Input: part model. Units: mm. Frame: model coordinates. A direction names the side the tool comes from. Round coordinates to 2 decimals unless told otherwise and drop trailing zeros. Loops run counter-clockwise (first coordinate to the right, second up) from the corner with the lowest first, then second, coordinate; pieces in that order, holes last. Notation, with made-up numbers: M 49.25,-5 L 98.25,-5 A21 ccw 98.25,11 Z; hole C 79,66.5 d1. An arc over 180 degrees is marked long. Use one line per item in the form item = value. Start each with the question number.
Q1. First-contact query: P1, Ø0.6, axis at x = 0, z = -7.5, coming from the +Y side; P2, Ø0.7, axis at y = -3.5, z = -5, coming from the -X side. Flat tips, straight axial feed; report the tip coordinate or a pass-through.
Q2. Ray query, line 1 along Y through (x, z) = (-0.45, -6.5); line 2 along Y through (x, z) = (0, -8); line 3 along Z through (x, y) = (0.05, 1.25). Return the intervals inside material, ascending.
Q3. Mould query, pull axis Y, two halves, no side actions, for faces 4 (the flat face through (0, -3, -4)), 5 (the flat face through (0.55, 3.5, -3.5)), 6 (the flat face through (0, 4.1, -4)). Classes: pulls with the +Y half, pulls with the -Y half, needs draft (parallel to the pull), parting line crosses it, or undercut.
Q4. Section query D-D, the plane y = 1.5. Output: boundary loops of the cut face in (x, z), and give its area (3 significant figures).
Q5. Section query A-A, the plane z = -1.5. Output: boundary loops of the cut face in (x, y).
Q6. Access query for faces 1 (the flat face through (-0.008, 3.694, -0.641)), 2 (the flat face through (-0.55, 3.5, -3.5)), 3 (the flat face through (0.55, -3.5, -3.5)). Directions: +Z, -Z, +X, -X, +Y, -Y. A direction counts if a zero-diameter tool reaches every point of the face in a straight line with its end or side. Return the directions, or none.
Q7. Section query B-B, the plane z = -6. Output: boundary loops of the cut face in (x, y), and give its area (3 significant figures).
```python
from build123d import *

# Parameters (mm, degrees)
F0_W         = 1.1
F0_H         = 7
F1_DEPTH     = 0.55
F2_W         = 0.7
F2_H         = 0.7
F3_DEPTH     = 1.2
F4_R         = 0.1
F7_DEPTH     = 0.45
F8_W         = 0.8
F8_H         = 0.8
F9_DEPTH     = 3
F10_R        = 0.1
F11_T1_DEPTH = 7.6228122918


# Not quite as in the source:
# - a fillet or chamfer that OpenCascade refuses, or shapes differently, is made with other operations: its cross-section is extruded or revolved along the edge and cut away or added


with BuildPart() as f1:
    # F0 (on Right) → F1 (new body, symmetric)
    with BuildSketch(Plane.YZ):
        with Locations((3.55, -3.5)):
            Rectangle(F0_W, F0_H)
    extrude(amount=F1_DEPTH, both=True)

    # F2 (on face) → F3 (join)
    with BuildSketch(Plane(origin=(0, 0, -7), x_dir=(1, 0, 0), z_dir=(0, 0, -1))):
        with Locations((0, -3.55)):
            Rectangle(F2_W, F2_H)
    extrude(amount=F3_DEPTH)

    # F4
    f4_edges = [f1.edges().sort_by_distance(p)[0] for p in [
        (0.55, 4.1, -3.5),
        (0.55, 3, -3.5),
        (-0.55, 4.1, -3.5),
        (0.35, 3.9, -7.6),
        (-0.35, 3.9, -7.6),
        (0.35, 3.2, -7.6),
        (-0.35, 3.2, -7.6),
        (-0.55, 3, -3.5),
    ]]
    fillet(f4_edges, radius=F4_R)

    # F6 (on mid) → F7 (join, symmetric)
    with BuildSketch(Plane(origin=(0, 3.55, 0), x_dir=(-1, 0, 0), z_dir=(0, 1, 0))):
        with BuildLine():
            ThreePointArc((0.4914213562, -8.1414213562), (0.4265366865, -8.1847759065), (0.35, -8.2))
            Line((0.35, -8.2), (-0.35, -8.2))
            ThreePointArc((-0.35, -8.2), (-0.4265366865, -8.1847759065), (-0.4914213562, -8.1414213562))
            Line((-0.4914213562, -8.1414213562), (-0.6328427125, -8))
            Line((-0.6328427125, -8), (-0.9863961031, -8.3535533906))
            Line((-0.9863961031, -8.3535533906), (-0.8449747468, -8.4949747468))
            ThreePointArc((-0.8449747468, -8.4949747468), (-0.6178784027, -8.6467156728), (-0.35, -8.7))
            Line((-0.35, -8.7), (0.35, -8.7))
            ThreePointArc((0.35, -8.7), (0.6178784027, -8.6467156728), (0.8449747468, -8.4949747468))
            Line((0.8449747468, -8.4949747468), (0.9863961031, -8.3535533906))
            Line((0.9863961031, -8.3535533906), (0.6328427125, -8))
            Line((0.6328427125, -8), (0.4914213562, -8.1414213562))
        make_face()
    extrude(amount=F7_DEPTH, both=True)

    # F8 (on face) → F9 (join, through all)
    with BuildSketch(Plane.XZ.offset(-3)):
        with Locations((0, -5.8)):
            Rectangle(F8_W, F8_H)
    extrude(amount=F9_DEPTH)

    # F10
    f10_edges = [f1.edges().sort_by_distance(p)[0] for p in [
        (-0.4, 1.5, -5.4),
        (-0.4, 1.5, -6.2),
        (0.4, 1.5, -6.2),
        (0.4, 1.5, -5.4),
    ]]
    fillet(f10_edges, radius=F10_R)

    # F11: chamfer of 0.8 x 1.3 on 1 edges, made by hand

    # F11_s2 → F11_t1 (cut)
    with BuildSketch(Plane.YZ.offset(-3.8114061459)):
        Polygon((3.3, 0), (4.1, -1.3), (4.1, 0), align=None)
    extrude(amount=F11_T1_DEPTH, mode=Mode.SUBTRACT)

    # F12: F1 across plane


with BuildPart() as f1_1:
    add(f1.part)
    add(f1.part.mirror(Plane.XZ))


solid = f1_1.part
```
Results found:
q1.P1 = 3.9
q1.P2 = -0.55
q2.line_1 = -4.1 to -3, 3 to 4.1
q2.line_2 = -3.9 to -3.2, 3.2 to 3.9
q2.line_3 = -6.2 to -5.4
q3.face_4 = undercut
q3.face_5 = needs draft
q3.face_6 = pulls with the +Y half
q4.outline = M -0.4,-6.1 A0.1 ccw -0.3,-6.2 L 0.3,-6.2 A0.1 ccw 0.4,-6.1 L 0.4,-5.5 A0.1 ccw 0.3,-5.4 L -0.3,-5.4 A0.1 ccw -0.4,-5.5 Z
q4.area = 0.631 mm²
q5.outline = M -0.55,-4 A0.1 ccw -0.45,-4.1 L 0.45,-4.1 A0.1 ccw 0.55,-4 L 0.55,-3.1 A0.1 ccw 0.45,-3 L -0.45,-3 A0.1 ccw -0.55,-3.1 Z; M -0.55,3.1 A0.1 ccw -0.45,3 L 0.45,3 A0.1 ccw 0.55,3.1 L 0.55,4 A0.1 ccw 0.45,4.1 L -0.45,4.1 A0.1 ccw -0.55,4 Z
q6.face_1 = +Z, +X, -X, +Y
q6.face_2 = +Z, -X, +Y, -Y
q6.face_3 = +Z, +X, +Y, -Y
q7.outline = M -0.55,-4 A0.1 ccw -0.45,-4.1 L 0.45,-4.1 A0.1 ccw 0.55,-4 L 0.55,-3.1 A0.1 ccw 0.45,-3 L 0.4,-3 L 0.4,3 L 0.45,3 A0.1 ccw 0.55,3.1 L 0.55,4 A0.1 ccw 0.45,4.1 L -0.45,4.1 A0.1 ccw -0.55,4 L -0.55,3.1 A0.1 ccw -0.45,3 L -0.4,3 L -0.4,-3 L -0.45,-3 A0.1 ccw -0.55,-3.1 Z
q7.area = 7.20 mm²
